```python
from build123d import *

# Parameters (mm, degrees)
SALIENTE_EXTRUIR1_DEPTH = 1.5


with BuildPart() as part:
    # Croquis1 → Saliente-Extruir1 (new body)
    with BuildSketch(Plane(origin=(0, 0, 0), x_dir=(-1, 0, 0), z_dir=(0, 0, -1))):
        with BuildLine():
            Line((18, 17.75), (14.25, 17.75))
            Line((14.25, 17.75), (14.25, 19.5))
            Line((14.25, 19.5), (4.5, 19.5))
            Line((4.5, 19.5), (4.5, 17.75))
            Line((4.5, 17.75), (-4.5, 17.75))
            Line((-4.5, 17.75), (-4.5, 19.5))
            Line((-4.5, 19.5), (-14.25, 19.5))
            Line((-14.25, 19.5), (-14.25, 17.75))
            Line((-14.25, 17.75), (-18, 17.75))
            ThreePointArc((-18, 17.75), (-19.414213562, 17.164213562), (-20, 15.75))
            Line((-20, 15.75), (-20, -15.75))
            ThreePointArc((-20, -15.75), (-19.414213562, -17.164213562), (-18, -17.75))
            Line((-18, -17.75), (-14.25, -17.75))
            Line((-14.25, -17.75), (-14.25, -19.5))
            Line((-14.25, -19.5), (-4.5, -19.5))
            Line((-4.5, -19.5), (-4.5, -17.75))
            Line((-4.5, -17.75), (4.5, -17.75))
            Line((4.5, -17.75), (4.5, -19.5))
            Line((4.5, -19.5), (14.25, -19.5))
            Line((14.25, -19.5), (14.25, -17.75))
            Line((14.25, -17.75), (18, -17.75))
            ThreePointArc((18, -17.75), (19.414213562, -17.164213562), (20, -15.75))
            Line((20, -15.75), (20, 15.75))
            ThreePointArc((20, 15.75), (19.414213562, 17.164213562), (18, 17.75))
        make_face()
        with BuildLine():
            Line((-0.596130775, -12.909090909), (-14.096130775, -8.693594715))
            ThreePointArc((-14.096130775, -8.693594715), (-15.111251307, -7.96935368), (-15.5, -6.784503806))
            Line((-15.5, -6.784503806), (-15.5, 6.784503806))
            ThreePointArc((-15.5, 6.784503806), (-15.111251307, 7.96935368), (-14.096130775, 8.693594715))
            Line((-14.096130775, 8.693594715), (-0.596130775, 12.909090909))
            ThreePointArc((-0.596130775, 12.909090909), (0, 13), (0.596130775, 12.909090909))
            Line((0.596130775, 12.909090909), (14.096130775, 8.693594715))
            ThreePointArc((14.096130775, 8.693594715), (15.111251307, 7.96935368), (15.5, 6.784503806))
            Line((15.5, 6.784503806), (15.5, -6.784503806))
            ThreePointArc((15.5, -6.784503806), (15.111251307, -7.96935368), (14.096130775, -8.693594715))
            Line((14.096130775, -8.693594715), (0.596130775, -12.909090909))
            ThreePointArc((0.596130775, -12.909090909), (0, -13), (-0.596130775, -12.909090909))
        make_face(mode=Mode.SUBTRACT)
    extrude(amount=-SALIENTE_EXTRUIR1_DEPTH)


solid = part.part
```
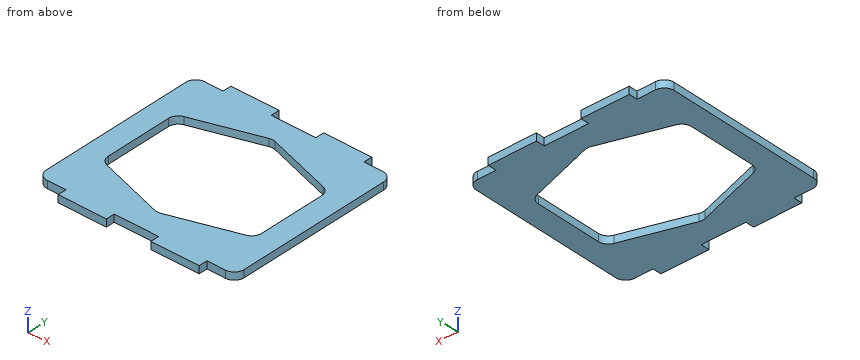
Here's how the part is built. I have some questions about the finished solid (model axes, mm). Give positions to 0.01 mm unless a question says otherwise; leave off trailing zeros. Order: outer loops, then holes, each group sorted by start corner. A loop starts at its lowest first (then second) coordinate and runs counter-clockwise, first axis right, second up. Notation, with made-up numbers: (-23.75, 82.25) - (-5.75, 82.25) arc R16 ccw to (-5.75, 94.25) - close; hole circle Ø8 at (-33.5, 28). An arc over 180 degrees is marked (long way). Answer as a JSON object with one key per item and string values. Group by question number.
Item 1: For P1, Ø0.8, axis at x = 15.5, z = 0.5, coming from the +Y side, with a flat end and sliding along its axis, tell me the tip position at first contact or that it passes through.
Item 2: Please list where these lines run through material, in increasing order: probe 1 along X at (y, z) = (-4.5, 0.25); probe 2 along Y at (x, z) = (-17.5, 0.95); probe 3 along Y at (x, z) = (-6.5, 0.25).
Item 3: If we section it at B-B on x = 13: Please give me the cut outline in (y, z), and give its area (3 significant figures).
Item 4: If we section it at A-A on y = 1.5: Please give me the cut outline in (x, z).
Result set:
{
 "1": {"P1": "y = 17.75"},
 "2": {"probe 1": "-20 to -15.5, 15.5 to 20", "probe 2": "-17.75 to 17.75", "probe 3": "-19.5 to -11.07, 11.07 to 19.5"},
 "3": {"outline": "(-19.5, 0) - (-9.04, 0) - (-9.04, 1.5) - (-19.5, 1.5) - close; (9.04, 0) - (19.5, 0) - (19.5, 1.5) - (9.04, 1.5) - close", "area": "31.4 mm²"},
 "4": {"outline": "(-20, 0) - (-15.5, 0) - (-15.5, 1.5) - (-20, 1.5) - close; (15.5, 0) - (20, 0) - (20, 1.5) - (15.5, 1.5) - close"}
}
